from build123d import *

# Parameters (mm, degrees)
SKETCH1_W           = 240
SKETCH1_H           = 240
SKETCH1_W_2         = 220
SKETCH1_H_2         = 220
BOSS_EXTRUDE1_DEPTH = 260
SKETCH2_W           = 240
SKETCH2_H           = 240
BOSS_EXTRUDE2_DEPTH = 10
SKETCH3_R           = 16.5
CUT_EXTRUDE1_DEPTH  = 20
CUT_EXTRUDE3_DEPTH  = 10
SKETCH8_W           = 100
SKETCH8_H           = 108.812952024
CUT_EXTRUDE4_DEPTH  = 296
BOSS_EXTRUDE4_DEPTH = 372
SKETCH10_W          = 200
SKETCH10_H          = 250
CUT_EXTRUDE5_DEPTH  = 372
SKETCH11_W          = 10
SKETCH11_H          = 220
BOSS_EXTRUDE6_DEPTH = 362
SKETCH12_W          = 70
SKETCH12_H          = 240
BOSS_EXTRUDE7_DEPTH = 10


with BuildPart() as part:
    # Sketch1 → Boss-Extrude1 (new body)
    with BuildSketch(Plane(origin=(0, 0, 0), x_dir=(1, 0, 0), z_dir=(0, 1, 0))):
        Rectangle(SKETCH1_W, SKETCH1_H)
        Rectangle(SKETCH1_W_2, SKETCH1_H_2, mode=Mode.SUBTRACT)
    extrude(amount=BOSS_EXTRUDE1_DEPTH)

    # Sketch2 → Boss-Extrude2 (add)
    with BuildSketch(Plane.XZ):
        Rectangle(SKETCH2_W, SKETCH2_H)
    extrude(amount=BOSS_EXTRUDE2_DEPTH)

    # Sketch3 → Cut-Extrude1 (cut)
    with BuildSketch(Plane.XZ.offset(10)):
        with Locations(Location((0, 0, 0), (0, 0, 270))):
            Circle(SKETCH3_R)
    extrude(amount=-CUT_EXTRUDE1_DEPTH, mode=Mode.SUBTRACT)

    # Sketch7 → Cut-Extrude3 (cut)
    with BuildSketch(Plane(origin=(0, -10, 0), x_dir=(-1, 0, 0), z_dir=(0, -1, 0))):
        with BuildLine():
            Line((-36.415999231, 33.587572106), (-35.001785669, 32.173358544))
            ThreePointArc((-35.001785669, 32.173358544), (-32.173358544, 32.173358544), (-32.173358544, 35.001785669))
            Line((-32.173358544, 35.001785669), (-33.587572106, 36.415999231))
            ThreePointArc((-33.587572106, 36.415999231), (-36.415999231, 36.415999231), (-36.415999231, 33.587572106))
        make_face()
        with BuildLine():
            Line((32.173358544, 35.001785669), (33.587572106, 36.415999231))
            ThreePointArc((33.587572106, 36.415999231), (36.415999231, 36.415999231), (36.415999231, 33.587572106))
            Line((36.415999231, 33.587572106), (35.001785669, 32.173358544))
            ThreePointArc((35.001785669, 32.173358544), (32.173358544, 32.173358544), (32.173358544, 35.001785669))
        make_face()
        with BuildLine():
            Line((35.001785669, -32.173358544), (36.415999231, -33.587572106))
            ThreePointArc((36.415999231, -33.587572106), (36.415999231, -36.415999231), (33.587572106, -36.415999231))
            Line((33.587572106, -36.415999231), (32.173358544, -35.001785669))
            ThreePointArc((32.173358544, -35.001785669), (32.173358544, -32.173358544), (35.001785669, -32.173358544))
        make_face()
        with BuildLine():
            Line((-36.415999231, -33.587572106), (-35.001785669, -32.173358544))
            ThreePointArc((-35.001785669, -32.173358544), (-32.173358544, -32.173358544), (-32.173358544, -35.001785669))
            Line((-32.173358544, -35.001785669), (-33.587572106, -36.415999231))
            ThreePointArc((-33.587572106, -36.415999231), (-36.415999231, -36.415999231), (-36.415999231, -33.587572106))
        make_face()
    extrude(amount=-CUT_EXTRUDE3_DEPTH, mode=Mode.SUBTRACT)

    # Sketch8 → Cut-Extrude4 (cut)
    with BuildSketch(Plane.XY.offset(120)):
        with Locations((0, 234.406476012)):
            Rectangle(SKETCH8_W, SKETCH8_H)
    extrude(amount=-CUT_EXTRUDE4_DEPTH, mode=Mode.SUBTRACT)

    # Sketch9 → Boss-Extrude4 (add)
    with BuildSketch(Plane(origin=(0, 260, 0), x_dir=(1, 0, 0), z_dir=(0, 1, 0))):
        Polygon((-50, 110), (-50, 120), (-120, 120), (-120, -120), (-50, -120), (-50, -110), (-110, -110), (-110, 110), align=None)
        Polygon((50, 110), (50, 120), (120, 120), (120, -120), (50, -120), (50, -110), (110, -110), (110, 110), align=None)
    extrude(amount=BOSS_EXTRUDE4_DEPTH)

    # Sketch10 → Cut-Extrude5 (cut)
    with BuildSketch(Plane(origin=(120, 0, 0), x_dir=(0, 0, -1), z_dir=(1, 0, 0))):
        with Locations((0, 135)):
            Rectangle(SKETCH10_W, SKETCH10_H)
    extrude(amount=-CUT_EXTRUDE5_DEPTH, mode=Mode.SUBTRACT)

    # Sketch11 → Boss-Extrude6 (add)
    with BuildSketch(Plane(origin=(0, 632, 0), x_dir=(1, 0, 0), z_dir=(0, 1, 0))):
        with Locations((55, 0)):
            Rectangle(SKETCH11_W, SKETCH11_H)
        with Locations((-55, 0)):
            Rectangle(SKETCH11_W, SKETCH11_H)
    extrude(amount=-BOSS_EXTRUDE6_DEPTH)

    # Sketch12 → Boss-Extrude7 (add)
    with BuildSketch(Plane.XZ.offset(-270)):
        with Locations((-85, 0)):
            Rectangle(SKETCH12_W, SKETCH12_H)
        with Locations((85, 0)):
            Rectangle(SKETCH12_W, SKETCH12_H)
    extrude(amount=BOSS_EXTRUDE7_DEPTH)


solid = part.part
Input: part model. Units: mm. Frame: model coordinates. A direction names the side the tool comes from. Coordinates: 2 decimals unless noted, no trailing zeros. Loops run counter-clockwise (first coordinate to the right, second up) from the corner with the lowest first, then second, coordinate; pieces in that order, holes last.
Q1. Cut plane D-D (x = 0). Output: boundary loops of the cut face in (y, z), then the cut area to 3 significant figures.
Q2. Material intervals for line 1 (X direction, y = 570, z = 65); line 2 (Z direction, x = 2, y = 107); line 3 (Y direction, x = -83, z = 51), sorted ascending.
Q3. Cut plane C-C (y = 57). Output: boundary loops of the cut face in (x, z), then the cut area to 3 significant figures.
Q4. Draft query along Z for faces 1 (the face through (-85, 448, 110)), 2 (the face through (-55, 315, 120)), 3 (the face through (-111, 632, 8)). Return one class per face: +Z half, -Z half, draft (parallel to the pull), parting line (faces both ways), or undercut.
Q5. Cut plane B-B (x = -66). Output: boundary loops of the cut face in (y, z), then the cut area to 3 significant figures.
Q6. Set-up query: faces 4 (the face through (2, 99, 110)), 5 (the face through (110, 448, 2)), 6 (the face through (-16.108, -5.07, 3.577)), 7 (the face through (50, 459, 2)). Return all of +Z, -Z, +X, -X, +Y, -Y with unobstructed straight access to the full face (end or side cutting, diameter ignored); none if empty.
Q7. Contact query for flat-ended pins moving along their axis: pin 1 (8 mm diameter, centred on x = -6.5, z = 117, fed in from +Y); pin 2 (12 mm diameter, centred on x = -29.5, z = 15, fed in from +Y). Output: stop coordinate, or through.
Q8. Cut plane A-A (z = -45). Output: boundary loops of the cut face in (x, y).
Working result:
1. outline: (-10, -120) - (180, -120) - (180, -110) - (0, -110) - (0, -16.5) - (-10, -16.5) - close; (-10, 16.5) - (0, 16.5) - (0, 110) - (180, 110) - (180, 120) - (-10, 120) - close
1. area: 5,670 mm2
2. line 1: x = -120 to -110, -60 to -50, 50 to 60, 110 to 120
2. line 2: z = -120 to -110, 110 to 120
2. line 3: y = -10 to 0, 260 to 270
3. outline: (-120, -120) - (120, -120) - (120, -100) - (110, -100) - (110, -110) - (-110, -110) - (-110, -100) - (-120, -100) - close; (-120, 100) - (-110, 100) - (-110, 110) - (110, 110) - (110, 100) - (120, 100) - (120, 120) - (-120, 120) - close
3. area: 5,200 mm2
4. face 1: undercut
4. face 2: +Z half
4. face 3: draft
5. outline: (-10, -120) - (632, -120) - (632, -110) - (270, -110) - (270, 110) - (632, 110) - (632, 120) - (-10, 120) - close; hole (0, -110) - (260, -110) - (260, 110) - (0, 110) - close
5. area: 17,200 mm2
6. face 4: none
6. face 5: +Y
6. face 6: +Y, -Y
6. face 7: +Z, -Z, +Y
7. pin 1: stops at y = 180
7. pin 2: stops at y = 0
8. outline: (-120, -10) - (120, -10) - (120, 10) - (110, 10) - (110, 0) - (-110, 0) - (-110, 10) - (-120, 10) - close; (-120, 260) - (-50, 260) - (-50, 632) - (-60, 632) - (-60, 270) - (-110, 270) - (-110, 632) - (-120, 632) - close; (50, 260) - (120, 260) - (120, 632) - (110, 632) - (110, 270) - (60, 270) - (60, 632) - (50, 632) - close
